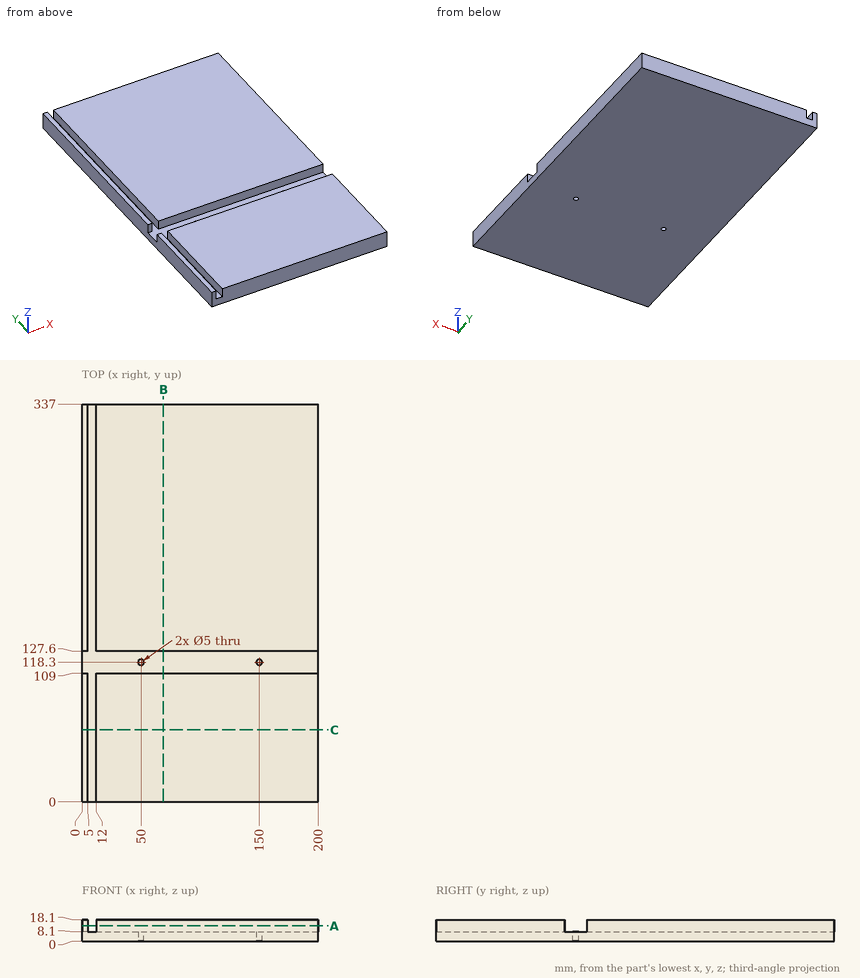
Print and shaded views of the part. All mm, measured from the part's lowest x, y and z. Round coordinates to 2 decimals unless told otherwise and drop trailing zeros. Loops run counter-clockwise (first coordinate to the right, second up) from the corner with the lowest first, then second, coordinate; pieces in that order, holes last. Notation, with made-up numbers: (44.5, -35) -> (83.5, -35) arc R11 ccw to (83.5, -25) -> close; hole circle Ø10 at (84.5, 12.25). An arc over 180 degrees is marked (long way). Use CSV: the item, a comma, the result in double quotes. Start each with the question number.
1) Cut at B-B, the plane x = 69. Write the cut outline in (y, z).
2) Cut at A-A, the plane z = 13. Write the cut outline in (x, y).
3) Drop a flat-ended pin along its axis: P1, Ø6.5, axis at x = 50, y = 118.3, coming from the +Z side. Give the stop position or say it passes through.
4) Wall check: L1, parallel to X at y = 118.3, z = 2; L2, parallel to Y at x = 184, z = 11.5; L3, parallel to X at y = 309, z = 10.25. Give the ranges that are in metal, low to high. Write a range as [from, to].
5) Cut at C-C, the plane y = 61. Write the cut outline in (x, z).
Determined:
1,outline,"(0, 0) -> (337, 0) -> (337, 18.1) -> (127.6, 18.1) -> (127.6, 8.1) -> (109, 8.1) -> (109, 18.1) -> (0, 18.1) -> close"
2,outline,"(0, 0) -> (5, 0) -> (5, 109) -> (0, 109) -> close; (0, 127.6) -> (5, 127.6) -> (5, 337) -> (0, 337) -> close; (12, 0) -> (200, 0) -> (200, 109) -> (12, 109) -> close; (12, 127.6) -> (200, 127.6) -> (200, 337) -> (12, 337) -> close"
3,P1,"stops at z = 8.1"
4,L1,"x = [0, 47.5], [52.5, 147.5], [152.5, 200]"
4,L2,"y = [0, 109], [127.6, 337]"
4,L3,"x = [0, 5], [12, 200]"
5,outline,"(0, 0) -> (200, 0) -> (200, 18.1) -> (12, 18.1) -> (12, 8.1) -> (5, 8.1) -> (5, 18.1) -> (0, 18.1) -> close"
